Read the model definition and answer for the solid it produces. Units are mm, in the model's axes. Face numbers are marked on the shaded views. A direction names the side the tool comes from. Round coordinates to 2 decimals unless told otherwise and drop trailing zeros. Write each loop counter-clockwise with the first axis right and the second up, starting at its lowest first coordinate (ties: lowest second). Pieces come first, ordered by that corner, then holes. Notation, with made-up numbers: (53.25, -19) - (66.25, -19) arc R23 cw to (66.25, 9) - close; hole circle Ø7 at (40, -7.75). An arc over 180 degrees is marked (long way). One line per item, written item: value. Start each with the question number.
(1) A flat-ended cylindrical pin translates along its axis: pin 1 Ø2.5 at (y, z) = (25, 0) entering from +X (3 decimals). Find the tip coordinate at first contact, or state that the pin passes through.
(2) A cutting plane is placed at B-B, the plane x = -4.25. Determine the outline of the cut face in (y, z), plus the area to 3 significant figures.
(3) For the marked faces 3 and 4, determine the directions among +Z, -Z, +X, -X, +Y, -Y from which every point of the face is accessible in a straight line to the end or side of a thin tool.
(4) A cutting plane is placed at A-A, the plane z = -4. Determine the outline of the cut face in (x, y).
(5) The mould has two halves that part along X. Classify the marked faces 1 and 2: +X half, -X half, draft (parallel to the pull), parting line (faces both ways), or undercut.
(6) A cutting plane is placed at C-C, the plane y = 86. Determine the outline of the cut face in (x, z).
(7) Find the intervals of material crossed by L1, parallel to Y at x = 9.3, z = 0; L2, parallel to Z at x = 4.5, y = 122; L3, parallel to X at y = 70.5, z = -1.5, in increasing order.
from build123d import *

# Parameters (mm, degrees)
SKETCH_1_W          = 20
SKETCH_1_H          = 15
SKETCH_1_W_2        = 18
SKETCH_1_H_2        = 13
EXTRUDE_1_DEPTH     = 305
SKETCH_2_R          = 1.45
CUT_EXTRUDE_1_DEPTH = 306.747035963
SKETCH_3_R          = 1.45
CUT_EXTRUDE_2_DEPTH = 306.532322349


with BuildPart() as part:
    # 草图1 → 拉伸-薄壁1 (new body)
    with BuildSketch(Plane(origin=(0, 0, 0), x_dir=(1, 0, 0), z_dir=(0, 1, 0))):
        Rectangle(SKETCH_1_W, SKETCH_1_H)
        Rectangle(SKETCH_1_W_2, SKETCH_1_H_2, mode=Mode.SUBTRACT)
    extrude(amount=EXTRUDE_1_DEPTH)

    # 草图2 → 切除-拉伸1 (cut, through all)
    with BuildSketch(Plane(origin=(10, 0, 0), x_dir=(0, 0, -1), z_dir=(1, 0, 0))):
        with Locations((0, 5)):
            Circle(SKETCH_2_R)
        with Locations((0, 25)):
            Circle(SKETCH_2_R)
    extrude(amount=-CUT_EXTRUDE_1_DEPTH, mode=Mode.SUBTRACT)

    # 草图3 → 切除-拉伸2 (cut, through all)
    with BuildSketch(Plane(origin=(0, 0, -7.5), x_dir=(-1, 0, 0), z_dir=(0, 0, -1))):
        with Locations((0, 15)):
            Circle(SKETCH_3_R)
        with Locations((0, 35)):
            Circle(SKETCH_3_R)
        with Locations((0, 55)):
            Circle(SKETCH_3_R)
    extrude(amount=-CUT_EXTRUDE_2_DEPTH, mode=Mode.SUBTRACT)


solid = part.part
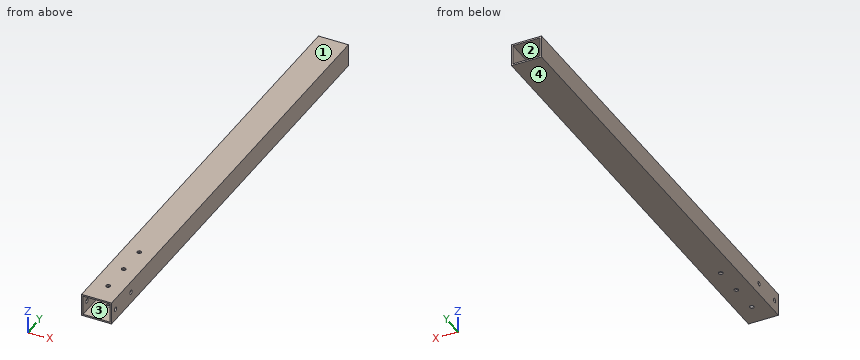
Here are the results:
1. pin 1: through
2. outline: (0, -7.5) - (305, -7.5) - (305, -6.5) - (0, -6.5) - close; (0, 6.5) - (305, 6.5) - (305, 7.5) - (0, 7.5) - close
2. area: 610 mm²
3. face 3: +Y, -Y
3. face 4: -Z, +X, -X, +Y, -Y
4. outline: (-10, 0) - (-9, 0) - (-9, 305) - (-10, 305) - close; (9, 0) - (10, 0) - (10, 305) - (9, 305) - close
5. face 1: draft
5. face 2: undercut
6. outline: (-10, -7.5) - (10, -7.5) - (10, 7.5) - (-10, 7.5) - close; hole (-9, -6.5) - (9, -6.5) - (9, 6.5) - (-9, 6.5) - close
7. L1: 0 to 3.55, 6.45 to 23.55, 26.45 to 305
7. L2: -7.5 to -6.5, 6.5 to 7.5
7. L3: -10 to -9, 9 to 10
